Input: part model. Units: mm. Frame: model coordinates. A direction names the side the tool comes from. Give positions to 0.01 mm unless a question says otherwise; leave off trailing zeros. Loops run counter-clockwise (first coordinate to the right, second up) from the corner with the lowest first, then second, coordinate; pieces in that order, holes last. Notation, with made-up numbers: M -29,50 L -6,50 A24 cw -6,72 Z; hole C 67.5,39 d7. An arc over 180 degrees is marked long. Use CSV: the item, a comma, the result in double quotes. Start each with the question number.
Q1. Pull-direction query (Y, two-part tool) for faces 1 (the flat face through (-3, -19.265, 2)), 2 (the flat face through (-0.686, 6, 12)), 3 (the cylindrical face through (5.383, 8.686, 2.465)); classes: released by +Y, released by -Y, zero draft, split by the parting line, or undercut.
Q2. Section C-C, the plane y = 12. Output: boundary loops of the cut face in (x, z).
Q3. Section B-B, the plane z = 2.25. Output: boundary loops of the cut face in (x, y), plus the area to 3 significant figures.
Q4. Pin query (flat end, axial travel): pin 1 (7.5 mm diameter, centred on x = -11, z = 9, fed in from -Y); pin 2 (8 mm diameter, centred on x = -9.5, z = 8, fed in from +Y); pin 3 (8 mm diameter, centred on y = 11, z = 9, fed in from -X); pin 4 (3.5 mm diameter, centred on x = -13.19, y = -11.76, fed in from -Z). Return the tip coordinate at first contact, or that it passes through.
Q5. Material intervals for line 1 along X through (y, z) = (10.5, 18.25); line 2 along Z through (x, y) = (-0.5, 9.5); line 3 along Y through (x, z) = (-13, 18.5), sorted ascending.
Q6. Section D-D, the plane x = 4. Output: boundary loops of the cut face in (y, z), plus the area to 3 significant figures.
Q7. Section A-A, the plane x = -2. Output: boundary loops of the cut face in (y, z), plus the area to 3 significant figures.
Q8. Reachability of faces 4 (the flat face through (-6, -1, 20)), 5 (the flat face through (-13, -0.265, 10)), 6 (the flat face through (-11, -4.265, 12)) from +Z, -Z, +X, -X, +Y, -Y: full face, straight path, thin tool, end or side. Return the list, or none.
from build123d import *

# Parameters (mm, degrees)
BOSS_EXTRUDE1_DEPTH = 5
BOSS_EXTRUDE2_DEPTH = 20
SKETCH3_W           = 20
SKETCH3_H           = 15
CUT_EXTRUDE1_DEPTH  = 21
SKETCH4_R           = 1.5
CUT_EXTRUDE2_DEPTH  = 21


with BuildPart() as part:
    # Sketch1 → Boss-Extrude1 (new body)
    with BuildSketch(Plane.XY):
        Polygon((14.31372549, -4.264705882), (34.31372549, -4.264705882), (34.31372549, -19.264705882), (-20.68627451, -19.264705882), (-20.68627451, -4.264705882), (-0.68627451, -4.264705882), (-0.68627451, 15.735294118), (14.31372549, 15.735294118), align=None)
    extrude(amount=BOSS_EXTRUDE1_DEPTH)

    # Sketch2 → Boss-Extrude2 (add)
    with BuildSketch(Plane(origin=(0, 0, 0), x_dir=(-1, 0, 0), z_dir=(0, 0, -1))):
        Polygon((0.68627451, 15.735294118), (4.68627451, 15.735294118), (4.68627451, -0.264705882), (6.079970528, -0.264705882), (20.68627451, -0.264705882), (20.68627451, -4.264705882), (0.68627451, -4.264705882), align=None)
    extrude(amount=-BOSS_EXTRUDE2_DEPTH)

    # Sketch3 → Cut-Extrude1 (cut, through all)
    with BuildSketch(Plane(origin=(0, 0, 0), x_dir=(-1, 0, 0), z_dir=(0, 0, -1))):
        with Locations((-24.31372549, -11.764705882)):
            Rectangle(SKETCH3_W, SKETCH3_H)
    extrude(amount=-CUT_EXTRUDE1_DEPTH, mode=Mode.SUBTRACT)

    # Sketch4 → Cut-Extrude2 (cut, through all)
    with BuildSketch(Plane(origin=(0, 0, 0), x_dir=(-1, 0, 0), z_dir=(0, 0, -1))):
        with Locations((-6.81372549, 8.235294118)):
            Circle(SKETCH4_R)
        with Locations((13.18627451, -11.764705882)):
            Circle(SKETCH4_R)
    extrude(amount=-CUT_EXTRUDE2_DEPTH, mode=Mode.SUBTRACT)


solid = part.part
A:
1,face 1,"released by -Y"
1,face 2,"zero draft"
1,face 3,"undercut"
2,outline,"M -4.69,0 L 14.31,0 L 14.31,5 L -0.69,5 L -0.69,20 L -4.69,20 Z"
3,outline,"M -20.69,-19.26 L 14.31,-19.26 L 14.31,15.74 L -4.69,15.74 L -4.69,-0.26 L -20.69,-0.26 Z; hole C -13.19,-11.76 d3; hole C 6.81,8.24 d3"
3,area,"955 mm^2"
4,pin 1,"y = -4.26"
4,pin 2,"y = -0.26"
4,pin 3,"x = -4.69"
4,pin 4,"z = 0"
5,line 1,"-4.69 to -0.69"
5,line 2,"0 to 5"
5,line 3,"-4.26 to -0.26"
6,outline,"M -19.26,0 L 15.74,0 L 15.74,5 L -19.26,5 Z"
6,area,"175 mm^2"
7,outline,"M -19.26,0 L 15.74,0 L 15.74,20 L -4.26,20 L -4.26,5 L -19.26,5 Z"
7,area,"475 mm^2"
8,face 4,"+Z, +X, -X, +Y, -Y"
8,face 5,"+Z, -Z, -X, +Y"
8,face 6,"+Z, +X, -X, -Y"
